Source: CAD feature listing. Evaluate the final solid. Frame: model axes, mm. A direction names the side the tool comes from. Round coordinates to 2 decimals unless told otherwise and drop trailing zeros. Order: outer loops, then holes, each group sorted by start corner. A loop starts at its lowest first (then second) coordinate and runs counter-clockwise, first axis right, second up. Notation, with made-up numbers: (-1, -1) -> (54, -1) arc R17 cw to (54, 26) -> close; hole circle Ø6 at (-4, 29.5). An arc over 180 degrees is marked (long way). Answer as CSV lines item,"result".
from build123d import *

# Parameters (mm, degrees)
F1_DEPTH = 2
F3_DEPTH = 2
F5_DEPTH = 10


with BuildPart() as f1:
    # F0 (on Top) → F1 (new body)
    with BuildSketch(Plane.XY):
        with BuildLine():
            Line((15.5, 38), (-15.5, 38))
            ThreePointArc((-15.5, 38), (-18.328427, 36.828427), (-19.5, 34))
            Line((-19.5, 34), (-19.5, -34))
            ThreePointArc((-19.5, -34), (-18.328427, -36.828427), (-15.5, -38))
            Line((-15.5, -38), (15.5, -38))
            ThreePointArc((15.5, -38), (18.328427, -36.828427), (19.5, -34))
            Line((19.5, -34), (19.5, 34))
            ThreePointArc((19.5, 34), (18.328427, 36.828427), (15.5, 38))
        make_face()
    extrude(amount=F1_DEPTH)

    # F2 (on face) → F3 (join)
    with BuildSketch(Plane.XY.offset(2)):
        with BuildLine():
            Line((19.5, -34), (19.5, 34))
            ThreePointArc((19.5, 34), (18.328427, 36.828427), (15.5, 38))
            Line((15.5, 38), (-15.5, 38))
            ThreePointArc((-15.5, 38), (-18.328427, 36.828427), (-19.5, 34))
            Line((-19.5, 34), (-19.5, -34))
            ThreePointArc((-19.5, -34), (-18.328427, -36.828427), (-15.5, -38))
            Line((-15.5, -38), (15.5, -38))
            ThreePointArc((15.5, -38), (18.328427, -36.828427), (19.5, -34))
        make_face()
        with BuildLine():
            ThreePointArc((-16.5, 34), (-16.207107, 34.707107), (-15.5, 35))
            Line((-15.5, 35), (15.5, 35))
            ThreePointArc((15.5, 35), (16.207107, 34.707107), (16.5, 34))
            Line((16.5, 34), (16.5, -34))
            ThreePointArc((16.5, -34), (16.207107, -34.707107), (15.5, -35))
            Line((15.5, -35), (-15.5, -35))
            ThreePointArc((-15.5, -35), (-16.207107, -34.707107), (-16.5, -34))
            Line((-16.5, -34), (-16.5, 34))
        make_face(mode=Mode.SUBTRACT)
    extrude(amount=F3_DEPTH)

    # F4 (on face) → F5 (join)
    with BuildSketch(Plane.XY.offset(2)):
        with BuildLine():
            ThreePointArc((-15.5, 38), (-18.328427, 36.828427), (-19.5, 34))
            Line((-19.5, 34), (-19.5, -34))
            ThreePointArc((-19.5, -34), (-18.328427, -36.828427), (-15.5, -38))
            Line((-15.5, -38), (15.5, -38))
            ThreePointArc((15.5, -38), (18.328427, -36.828427), (19.5, -34))
            Line((19.5, -34), (19.5, 34))
            ThreePointArc((19.5, 34), (18.328427, 36.828427), (15.5, 38))
            Line((15.5, 38), (-15.5, 38))
        make_face()
        with BuildLine():
            ThreePointArc((-18, 34), (-17.267767, 35.767767), (-15.5, 36.5))
            Line((-15.5, 36.5), (15.5, 36.5))
            ThreePointArc((15.5, 36.5), (17.267767, 35.767767), (18, 34))
            Line((18, 34), (18, -34))
            ThreePointArc((18, -34), (17.267767, -35.767767), (15.5, -36.5))
            Line((15.5, -36.5), (-15.5, -36.5))
            ThreePointArc((-15.5, -36.5), (-17.267767, -35.767767), (-18, -34))
            Line((-18, -34), (-18, 34))
        make_face(mode=Mode.SUBTRACT)
    extrude(amount=F5_DEPTH)


solid = f1.part
1. Section query B-B on y = -18. Return loops of the section in (x, z), and give its area (3 significant figures).
Results below:
outline,"(-19.5, 0) -> (19.5, 0) -> (19.5, 12) -> (18, 12) -> (18, 4) -> (16.5, 4) -> (16.5, 2) -> (-16.5, 2) -> (-16.5, 4) -> (-18, 4) -> (-18, 12) -> (-19.5, 12) -> close"
area,"114 mm2"
2. Pin query (flat end, axial travel): pin 1 (1.5 mm diameter, centred on x = 4, y = -2, fed in from +Z). Return the tip coordinate at first contact, or that it passes through.
Results below:
pin 1,"z = 2"
3. Reachability of faces 4 (the flat face through (0, 38, 6)), 5 (the flat face through (0, -35, 3)) from +Z, -Z, +X, -X, +Y, -Y: full face, straight path, thin tool, end or side. Return the list, or none.
Results below:
face 4,"+Z, -Z, +X, -X, +Y"
face 5,"+Z"
4. Section query C-C on x = 8. Return loops of the section in (y, z), and give its area (3 significant figures).
Results below:
outline,"(-38, 0) -> (38, 0) -> (38, 12) -> (36.5, 12) -> (36.5, 4) -> (35, 4) -> (35, 2) -> (-35, 2) -> (-35, 4) -> (-36.5, 4) -> (-36.5, 12) -> (-38, 12) -> close"
area,"188 mm2"
5. Section query A-A on z = 10.25. Return loops of the section in (x, y).
Results below:
outline,"(-19.5, -34) arc R4 ccw to (-15.5, -38) -> (15.5, -38) arc R4 ccw to (19.5, -34) -> (19.5, 34) arc R4 ccw to (15.5, 38) -> (-15.5, 38) arc R4 ccw to (-19.5, 34) -> close; hole (-18, -34) arc R2.5 ccw to (-15.5, -36.5) -> (15.5, -36.5) arc R2.5 ccw to (18, -34) -> (18, 34) arc R2.5 ccw to (15.5, 36.5) -> (-15.5, 36.5) arc R2.5 ccw to (-18, 34) -> close"
6. Line query: L1, parallel to Y at x = -15, z = 9; L2, parallel to X at y = 33, z = 10.25; L3, parallel to X at y = 30, z = 2.75. Output: solid intervals per line, ascending. Write a range as [from, to].
Results below:
L1,"[-38, -36.5], [36.5, 38]"
L2,"[-19.5, -18], [18, 19.5]"
L3,"[-19.5, -16.5], [16.5, 19.5]"
7. Mould query, pull axis X, two halves, no side actions, for faces 1 (the cylindrical face through (17, 36, 8)), 2 (the cylindrical face through (18.359, 36.797, 5.916)), 3 (the flat face through (0, -38, 6)). Classes: released by +X, released by -X, zero draft, split by the parting line, or undercut.
Results below:
face 1,"undercut"
face 2,"released by +X"
face 3,"zero draft"
